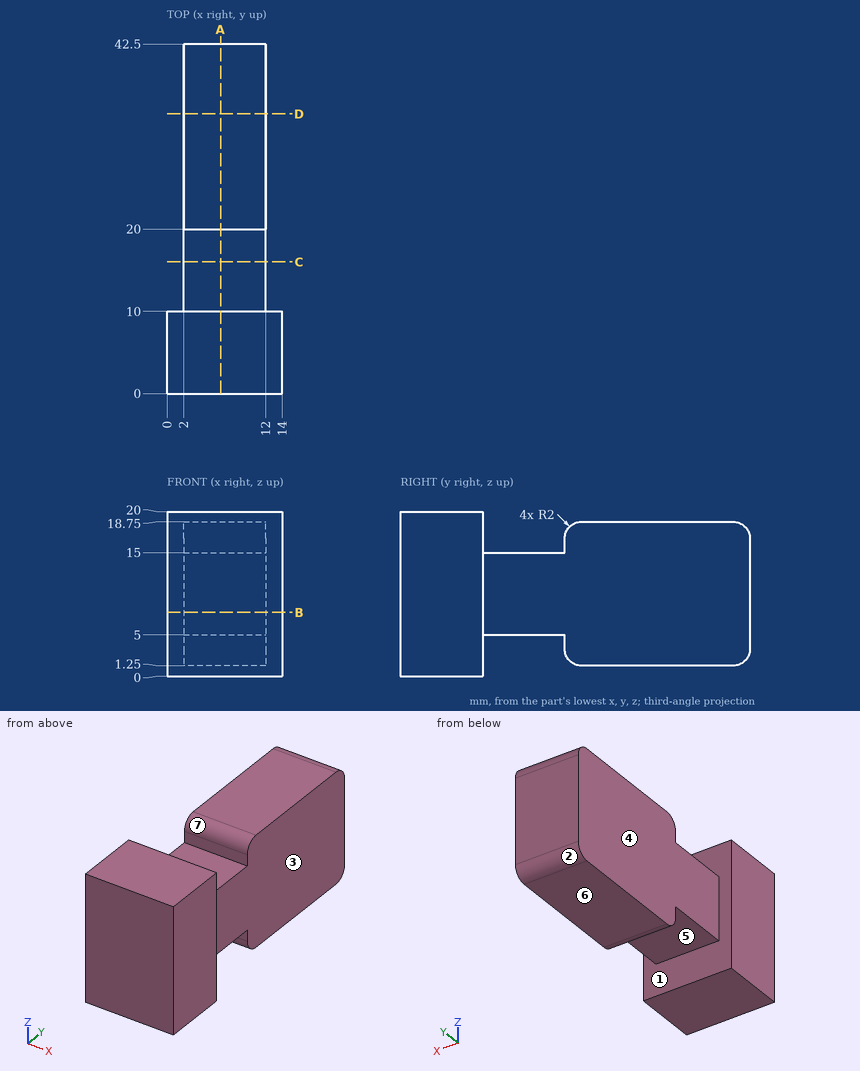
Geometry check sheet. Reference: drawing and pictorial views, mm from the part's lowest x, y, z. A direction names the side the tool comes from. Coordinates: 2 decimals unless noted, no trailing zeros. Order: outer loops, then holes, each group sorted by start corner. A loop starts at its lowest first (then second) coordinate and runs counter-clockwise, first axis right, second up.
Item 1: Material ranges on L1, parallel to Y at x = 8.25, z = 3.75; L2, parallel to X at y = 11, z = 11.5; L3, parallel to Z at x = 11.75, y = 19.5, recorded low to high.
Filled in:
L1: y = 0 to 10, 20 to 42.5
L2: x = 2 to 12
L3: z = 5 to 15
Item 2: Release check for a two-part mould opening along Y. For the marked faces 1, 2 and 3 record: +Y half, -Y half, draft (parallel to the pull), parting line (faces both ways), or undercut.
Filled in:
face 1: undercut
face 2: +Y half
face 3: draft
Item 3: Section check D-D, the plane y = 34. Enter the section's corners in (x, z), then the cut area to 3 significant figures.
Filled in:
outline: (2, 1.25) - (12, 1.25) - (12, 18.75) - (2, 18.75) - close
area: 175 mm2
Item 4: Section check C-C, the plane y = 16. Enter the section's corners in (x, z), then the cut area to 3 significant figures.
Filled in:
outline: (2, 5) - (12, 5) - (12, 15) - (2, 15) - close
area: 100 mm2
Item 5: Access from +Z, -Z, +X, -X, +Y, -Y to the whole of each face (thin tool, end or side, straight path). Record for the marked faces 4, 5, 6 and 7.
Filled in:
face 4: +Z, -Z, -X, +Y
face 5: -Z, +X, -X
face 6: -Z, +X, -X, +Y
face 7: +Z, +X, -X
Item 6: Depth check by flat-ended pin: pin 1 (4 mm diameter, centred on y = 21, z = 16.5, fed in from +X); pin 2 (1 mm diameter, centred on x = 11, y = 31, fed in from +Z); pin 3 (6 mm diameter, centred on y = 20, z = 4.5, fed in from -X). Enter the tip coordinate at first touch or a pass-through.
Filled in:
pin 1: stops at x = 12
pin 2: stops at z = 18.75
pin 3: stops at x = 2
Item 7: Section check B-B, the plane z = 7.75. Enter the section's corners in (x, y), then the cut area to 3 significant figures.
Filled in:
outline: (0, 0) - (14, 0) - (14, 10) - (12, 10) - (12, 42.5) - (2, 42.5) - (2, 10) - (0, 10) - close
area: 465 mm2
Item 8: Section check A-A, the plane x = 6.5. Enter the section's corners in (y, z), then the cut area to 3 significant figures.
Filled in:
outline: (0, 0) - (10, 0) - (10, 5) - (20, 5) - (20, 3.25) arc R2 ccw to (22, 1.25) - (40.5, 1.25) arc R2 ccw to (42.5, 3.25) - (42.5, 16.75) arc R2 ccw to (40.5, 18.75) - (22, 18.75) arc R2 ccw to (20, 16.75) - (20, 15) - (10, 15) - (10, 20) - (0, 20) - close
area: 690 mm2
